```python
from build123d import *


with BuildPart() as f1:
    # F0 (on Front) → F1 (revolve)
    with BuildSketch(Plane.XZ):
        with BuildLine():
            Line((0, 38.1), (0, 0))
            Line((0, 0), (14.2875, 0))
            ThreePointArc((14.2875, 0), (13.899108, 1.521657), (12.828956, 2.671031))
            Line((12.828956, 2.671031), (7.631716, 6.010877))
            ThreePointArc((7.631716, 6.010877), (6.623452, 7.052022), (6.182959, 8.4328))
            Line((6.182959, 8.4328), (3.8481, 38.1))
            ThreePointArc((3.8481, 38.1), (3.846534, 38.139857), (3.8481, 38.179714))
            ThreePointArc((3.8481, 38.179714), (3.39398, 38.645156), (2.854139, 38.282619))
            ThreePointArc((2.854139, 38.282619), (2.762666, 38.150718), (2.610375, 38.1))
            Line((2.610375, 38.1), (0, 38.1))
        make_face()
    revolve(axis=Axis((0, 0, 19.05), (0, 0, 1)))


solid = f1.part
```
Design review of the part built by this model. Coordinates are the model's own, in mm. Give positions to 0.01 mm unless a question says otherwise; leave off trailing zeros. Loops run counter-clockwise (first coordinate to the right, second up) from the corner with the lowest first, then second, coordinate; pieces in that order, holes last. Notation, with made-up numbers: M 37,56.25 L 43,56.25 A26 cw 43,75.25 Z; hole C 19.25,89 d11. An arc over 180 degrees is marked long. Return JSON: item names as keys, results as strings. Group by question number.
Item 1: We need section C-C (z = 14). Give the boundary of the cut face in (x, y), and give its area (3 significant figures).
Item 2: We need section D-D (z = 5.5). Give the boundary of the cut face in (x, y), and give its area (3 significant figures).
Item 3: Insertion check: pin 1 Ø8 at (y, z) = (10, 32) entering from +X; pin 2 Ø10 at (x, z) = (1.5, 5.5) entering from -Y; pin 3 Ø5 at (x, z) = (5.5, 10.5) entering from +Y; pin 4 Ø12 at (y, z) = (10, 16.5) entering from +X. Each pin has a flat end and moves straight along its axis. Give the tip position at first contact, or say it passes through.
Item 4: Mouldability with a two-part tool opening along Y and no side actions: class faces 1 (the conical face through (-6.257, -4.797, 5.849)), 2 (the flat face through (0, 0, 0)), 3 (the flat face through (0, 0, 38.1)) as released by +Y, released by -Y, zero draft, split by the parting line, or undercut.
Item 5: For probe 1 along Z at (x, y) = (1.5, 7.5); probe 2 along Y at (x, z) = (-1.75, 17.5); probe 3 along Z at (x, y) = (8.75, 3.5), list the stretches that pass through material, from the lowest coordinate up.
Output:
{
 "1": {"outline": "C 0,0 d11.49", "area": "104 mm^2"},
 "2": {"outline": "C 0,0 d16.85", "area": "223 mm^2"},
 "3": {"pin 1": "passes through", "pin 2": "stops at y = -14.22", "pin 3": "stops at y = 5.24", "pin 4": "stops at x = 3.88"},
 "4": {"face 1": "split by the parting line", "face 2": "zero draft", "face 3": "undercut"},
 "5": {"probe 1": "z = 0 to 6", "probe 2": "y = -5.18 to 5.18", "probe 3": "z = 0 to 4.86"}
}
